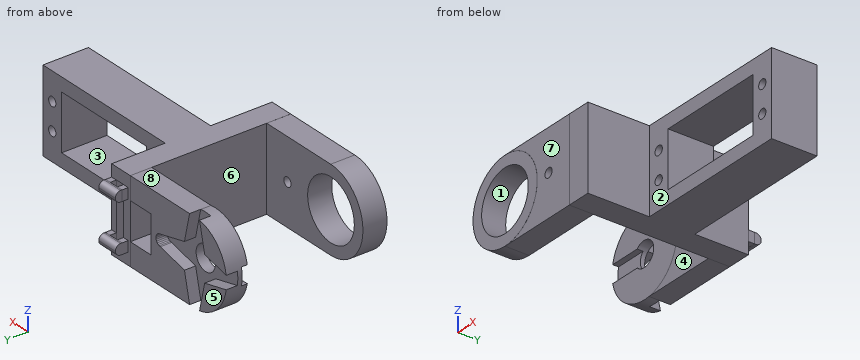
```python
from build123d import *

# Parameters (mm, degrees)
SKETCH002_W     = 8.977869
SKETCH002_H     = 59.983136
PAD001_DEPTH    = 15.5
SKETCH003_W     = 3.492328
SKETCH003_H     = 22.021174
POCKET001_DEPTH = 3
FILLET_R        = 2
FILLET001_R     = 2
SKETCH004_W     = 2.246188
SKETCH004_H     = 3.944797
SKETCH004_W_2   = 2.255042
SKETCH004_H_2   = 3.950065
PAD002_DEPTH    = 2.3
SKETCH007_W     = 7.994439
SKETCH007_H     = 30.992103
PAD004_DEPTH    = 28.65
SKETCH008_R     = 15.649013
PAD005_DEPTH    = 8
SKETCH009_W     = 10.023189
SKETCH009_H     = 13.999053
POCKET002_DEPTH = 8.001
POCKET003_DEPTH = 4.18
SKETCH011_R     = 4.641628
POCKET004_DEPTH = 5
POCKET007_DEPTH = 2.2
SKETCH012_W     = 8.980885
SKETCH012_H     = 30.993558
PAD006_DEPTH    = 31
SKETCH013_R     = 15.496795
PAD007_DEPTH    = 9
SKETCH014_R     = 11.256607
POCKET005_DEPTH = 9.001
SKETCH015_R     = 1.740109
POCKET006_DEPTH = 9.001
SKETCH006_W     = 2.5
SKETCH006_H     = 3.94941
EXTRUDE_DEPTH   = 8
FILLET003_R     = 1.97
SKETCH005_W     = 2.501053
SKETCH005_H     = 3.940234
PAD003_DEPTH    = 8
FILLET002_R     = 1.97
SKETCH_W        = 58.960041
SKETCH_H        = 16.989173
PAD_DEPTH       = 15.5
SKETCH001_R     = 1.754684
SKETCH001_R_2   = 1.752789
SKETCH001_W     = 40.995754
SKETCH001_H     = 20.714458
POCKET_DEPTH    = 16.990173


with BuildPart() as obj1:
    # Sketch002 → Pad001 (new body, symmetric)
    with BuildSketch(Plane.XY):
        with Locations((31.5110655, -25.991567)):
            Rectangle(SKETCH002_W, SKETCH002_H)
    extrude(amount=PAD001_DEPTH, both=True)

    # Sketch003 (on Face1 of Pad001) → Pocket001 (cut)
    with BuildSketch(Plane(origin=(0, 4.000001, 0), x_dir=(-1, 0, 0), z_dir=(0, 1, 0))):
        with Locations((-32.0097, 0.009076)):
            Rectangle(SKETCH003_W, SKETCH003_H)
    extrude(amount=-POCKET001_DEPTH, mode=Mode.SUBTRACT)

    # Fillet
    fillet_edges = [obj1.edges().sort_by_distance(p)[0] for p in [
        (32.0097, 1.000001, -11.001511),
    ]]
    fillet(fillet_edges, radius=FILLET_R)

    # Fillet001
    fillet001_edges = [obj1.edges().sort_by_distance(p)[0] for p in [
        (32.0097, 1.000001, 11.019663),
    ]]
    fillet(fillet001_edges, radius=FILLET001_R)

    # Sketch004 (on Face7 of Fillet001) → Pad002 (join)
    with BuildSketch(Plane(origin=(0, 4.000001, 0), x_dir=(-1, 0, 0), z_dir=(0, 1, 0))):
        with Locations((-34.878453, -8.9877845)):
            Rectangle(SKETCH004_W, SKETCH004_H)
        with Locations((-29.13443, -9.0147575)):
            Rectangle(SKETCH004_W_2, SKETCH004_H_2)
        with Locations((-34.878453, 8.9877845)):
            Rectangle(SKETCH004_W, SKETCH004_H)
        with Locations((-29.13443, 9.0147575)):
            Rectangle(SKETCH004_W_2, SKETCH004_H_2)
    extrude(amount=PAD002_DEPTH)


with BuildPart() as parte_arriba_motor:
    # Sketch007 (on Face1 of CopyPad004) → Pad004 (new body)
    with BuildSketch(Plane(origin=(27.022131, 0, 0), x_dir=(0, -1, 0), z_dir=(-1, 0, 0))):
        with Locations((-0.0007855, 0.0019735)):
            Rectangle(SKETCH007_W, SKETCH007_H)
    extrude(amount=PAD004_DEPTH)

    # Sketch008 (on Face3 of Pad004) → Pad005 (join)
    with BuildSketch(Plane(origin=(0, 3.998005, 0), x_dir=(-1, 0, 0), z_dir=(0, 1, 0))):
        with Locations((3.815743, 0.001435)):
            Circle(SKETCH008_R)
    extrude(amount=-PAD005_DEPTH)

    # Sketch009 (on Face9 of Pad005) → Pocket002 (cut, through all)
    with BuildSketch(Plane(origin=(0, 3.998005, 0), x_dir=(-1, 0, 0), z_dir=(0, 1, 0))):
        with Locations((-22.0115905, -0.0004715)):
            Rectangle(SKETCH009_W, SKETCH009_H)
    extrude(amount=-POCKET002_DEPTH, mode=Mode.SUBTRACT)

    # Sketch010 (on Face12 of Pocket002) → Pocket003 (cut)
    with BuildSketch(Plane(origin=(0, 3.998005, 0), x_dir=(-1, 0, 0), z_dir=(0, 1, 0))):
        Polygon((-0.879047, 4.879039), (-12.499996, 2.15), (-13.056458, 2.076739), (-13.574997, 1.861954), (-14.020602, 1.519604), (-14.361478, 1.075023), (-14.576989, 0.55653), (-14.649981, 0), (-14.576447, -0.556616), (-14.361427, -1.07512), (-14.019322, -1.51973), (-13.575246, -1.861696), (-13.056714, -2.076535), (-12.500516, -2.149443), (-0.879091, -4.879015), (1.6565, -15.670952), (4.613011, -15.847545), (6.390335, -15.545628), (8.879035, -4.879036), (19.292059, -2.465662), (19.451073, -1.246381), (19.49725, -0.017855), (19.447609, 1.211716), (19.306059, 2.428864), (8.879012, 4.879032), (6.402977, 15.480504), (4.635699, 15.800562), (1.61602, 15.605743), align=None)
    extrude(amount=-POCKET003_DEPTH, mode=Mode.SUBTRACT)

    # Sketch011 (on Face14 of Pocket003) → Pocket004 (cut)
    with BuildSketch(Plane(origin=(0, -0.181995, 0), x_dir=(-1, 0, 0), z_dir=(0, 1, 0))):
        with Locations((3.991006, 0)):
            Circle(SKETCH011_R)
    extrude(amount=-POCKET004_DEPTH, mode=Mode.SUBTRACT)

    # Sketch016 (on Face20 of Pocket004) → Pocket007 (cut)
    with BuildSketch(Plane.XZ.offset(4.001995)):
        Polygon((-19.274756, 3.229076), (-19.698963, 0), (-19.323395, -3.255331), (-6.564783, -3.255331), (-7.508081, -1.875622), (-7.786129, -0.643242), (-7.892649, 0.261497), (-7.606458, 1.237008), (-7.387746, 2.244735), (-6.500566, 3.229076), align=None)
    extrude(amount=-POCKET007_DEPTH, mode=Mode.SUBTRACT)


with BuildPart() as parte_abajo_motor:
    # Sketch012 (on Face1 of CopyPad005) → Pad006 (new body)
    with BuildSketch(Plane(origin=(27.022131, 0, 0), x_dir=(0, -1, 0), z_dir=(-1, 0, 0))):
        with Locations((51.4901415, -0.003249)):
            Rectangle(SKETCH012_W, SKETCH012_H)
    extrude(amount=PAD006_DEPTH)

    # Sketch013 (on Face4 of Pad006) → Pad007 (join)
    with BuildSketch(Plane(origin=(0, -46.999699, 0), x_dir=(-1, 0, 0), z_dir=(0, 1, 0))):
        with Locations((3.931386, -0.003132)):
            Circle(SKETCH013_R)
    extrude(amount=-PAD007_DEPTH)

    # Sketch014 (on Face8 of Pad007) → Pocket005 (cut, through all)
    with BuildSketch(Plane(origin=(0, -46.999699, 0), x_dir=(-1, 0, 0), z_dir=(0, 1, 0))):
        with Locations((4.019337, -0.005181)):
            Circle(SKETCH014_R)
    extrude(amount=-POCKET005_DEPTH, mode=Mode.SUBTRACT)

    # Sketch015 (on Face2 of Pocket005) → Pocket006 (cut, through all)
    with BuildSketch(Plane(origin=(0, -46.999699, 0), x_dir=(-1, 0, 0), z_dir=(0, 1, 0))):
        with Locations((-17.01331, 0.008823)):
            Circle(SKETCH015_R)
    extrude(amount=-POCKET006_DEPTH, mode=Mode.SUBTRACT)


with BuildPart() as fillet003:
    # Sketch006 (on Face1 of CopyPad003) → Extrude (new body)
    with BuildSketch(Plane(origin=(28.006909, 0, 0), x_dir=(0, -1, 0), z_dir=(-1, 0, 0))):
        with Locations((-7.549415, 9.015147)):
            Rectangle(SKETCH006_W, SKETCH006_H)
    extrude(amount=EXTRUDE_DEPTH)


with BuildPart() as fillet003_1:
    # Extrude placement: moved
    add(fillet003.part.moved(Location((8.02, 0, 0))))

    # Fillet003
    fillet003_edges = [fillet003_1.edges().sort_by_distance(p)[0] for p in [
        (32.026909, 8.799415, 10.989852),
        (32.026909, 8.799415, 7.040442),
    ]]
    fillet(fillet003_edges, radius=FILLET003_R)


with BuildPart() as obj2:
    # Sketch005 (on Face1 of CopyPad002) → Pad003 (new body)
    with BuildSketch(Plane(origin=(28.006909, 0, 0), x_dir=(0, -1, 0), z_dir=(-1, 0, 0))):
        with Locations((-7.5503545, -9.00987)):
            Rectangle(SKETCH005_W, SKETCH005_H)
    extrude(amount=-PAD003_DEPTH)

    # Fillet002
    fillet002_edges = [obj2.edges().sort_by_distance(p)[0] for p in [
        (32.006909, 8.800881, -7.039753),
        (32.006909, 8.800881, -10.979987),
    ]]
    fillet(fillet002_edges, radius=FILLET002_R)

    # Fusion: union Fillet003
    add(fillet003_1.part)


with BuildPart() as obj3:
    # Sketch → Pad (new body, symmetric)
    with BuildSketch(Plane.XY):
        with Locations((65.4798945, -24.5020905)):
            Rectangle(SKETCH_W, SKETCH_H)
    extrude(amount=PAD_DEPTH, both=True)

    # Sketch001 (on Face1 of Pad) → Pocket (cut, through all)
    with BuildSketch(Plane(origin=(0, -16.007504, 0), x_dir=(-1, 0, 0), z_dir=(0, 1, 0))):
        with Locations((-90.493328, 5.048292)):
            Circle(SKETCH001_R)
        with Locations((-90.493328, -5.048292)):
            Circle(SKETCH001_R)
        with Locations((-40.494466, 5.040685)):
            Circle(SKETCH001_R_2)
        with Locations((-40.494466, -5.040685)):
            Circle(SKETCH001_R_2)
        with Locations((-65.495859, 0.000125)):
            Rectangle(SKETCH001_W, SKETCH001_H)
    extrude(amount=-POCKET_DEPTH, mode=Mode.SUBTRACT)

    # Fusion001: union obj1, parte_arriba_motor, parte_abajo_motor, obj2
    add(obj1.part)
    add(parte_arriba_motor.part)
    add(parte_abajo_motor.part)
    add(obj2.part)


solid = obj3.part
```
Here's how the part is built. I have some questions about the finished solid (model axes, mm). Face numbers are marked on the shaded views. A direction names the side the tool comes from. Round coordinates to 2 decimals unless told otherwise and drop trailing zeros. Write each loop counter-clockwise with the first axis right and the second up, starting at its lowest first coordinate (ties: lowest second). Pieces come first, ordered by that corner, then holes.
Q1. If we mould it in two halves opening along Y, with no side actions, what happens to the marked faces 5, 6, 7 and 8? For each: +Y half, -Y half, draft (parallel to the pull), parting line (faces both ways), or undercut.
Q2. If we section it at B-B on y = -35: Write out the boundary of the cut face in (x, z).
Q3. Will these pins go through, and if not, where does the flat tip stop? P1, Ø10, axis at x = 32, z = 5, coming from the -Y side; P2, Ø2.5, axis at y = 5, z = -9, coming from the +X side; P3, Ø18.5, axis at y = -24.5, z = -0.5, coming from the -X side.
Q4. Which directions (+Z, -Z, +X, -X, +Y, -Y) give clear straight access to the entire face, cutting with the end or side of a thin tool? Please do the marked faces 1, 2, 3 and 4.
Q5. Please list where these lines run through material, in increasing order: probe 1 along X at (y, z) = (-1, 0); probe 2 along Y at (x, z) = (15, 7); probe 3 along Y at (x, z) = (-6, 12.5).
Answer below:
1. face 5: +Y half
1. face 6: undercut
1. face 7: -Y half
1. face 8: draft
2. outline: (27.02, -15.5) - (36, -15.5) - (36, 15.5) - (27.02, 15.5) - close
3. P1: stops at y = -55.98
3. P2: stops at x = 36
3. P3: stops at x = 27.02
4. face 1: -Y
4. face 2: +Z, -Z, +X, -Y
4. face 3: +Y, -Y
4. face 4: +Z, -Z, -X
5. probe 1: x = -19.46 to -8.63, 0.65 to 17, 27.02 to 36
5. probe 2: y = -55.98 to -47, -4 to 4
5. probe 3: y = -56 to -47, -4 to -0.18
